```python
from build123d import *

# Parameters (mm, degrees)
SKETCH_1_R          = 3
EXTRUDE_1_DEPTH     = 3
CHAMFER_1_SIZE      = 0.2
SKETCH_2_OUTSIDE_W  = 22.662
SKETCH_2_OUTSIDE_H  = 21.114
SKETCH_2_OUTSIDE_R  = 5
CUT_EXTRUDE_1_DEPTH = 3
CUT_EXTRUDE_1_TAPER = 45
SKETCH_3_OUTSIDE_W  = 22.662
SKETCH_3_OUTSIDE_H  = 21.114
SKETCH_3_OUTSIDE_R  = 5
CUT_EXTRUDE_2_DEPTH = 3
CUT_EXTRUDE_2_TAPER = 45


with BuildPart() as part:
    # Эскиз1 → Бобышка-Вытянуть1 (new body)
    with BuildSketch(Plane.XY):
        Polygon((5.773502692, 0), (2.886751346, 5), (-2.886751346, 5), (-5.773502692, 0), (-2.886751346, -5), (2.886751346, -5), align=None)
        Circle(SKETCH_1_R, mode=Mode.SUBTRACT)
    extrude(amount=EXTRUDE_1_DEPTH)

    # Фаска1
    chamfer_1_edges = [part.edges().sort_by_distance(p)[0] for p in [
        (-3, 0, 0),
        (-3, 0, 3),
    ]]
    chamfer(chamfer_1_edges, length=CHAMFER_1_SIZE)

    # Эскиз2 outside → Вырез-Вытянуть1 (cut)
    with BuildSketch(Plane.XY.offset(3)):
        Rectangle(SKETCH_2_OUTSIDE_W, SKETCH_2_OUTSIDE_H)
        Circle(SKETCH_2_OUTSIDE_R, mode=Mode.SUBTRACT)
    extrude(amount=-CUT_EXTRUDE_1_DEPTH, taper=CUT_EXTRUDE_1_TAPER, mode=Mode.SUBTRACT)

    # Эскиз3 outside → Вырез-Вытянуть2 (cut)
    with BuildSketch(Plane(origin=(0, 0, 0), x_dir=(-1, 0, 0), z_dir=(0, 0, -1))):
        Rectangle(SKETCH_3_OUTSIDE_W, SKETCH_3_OUTSIDE_H)
        Circle(SKETCH_3_OUTSIDE_R, mode=Mode.SUBTRACT)
    extrude(amount=-CUT_EXTRUDE_2_DEPTH, taper=CUT_EXTRUDE_2_TAPER, mode=Mode.SUBTRACT)


solid = part.part
```
Input: part model. Units: mm. Frame: model coordinates. Give positions to 0.01 mm unless a question says otherwise; leave off trailing zeros. Order: outer loops, then holes, each group sorted by start corner. A loop starts at its lowest first (then second) coordinate and runs counter-clockwise, first axis right, second up. Notation, with made-up numbers: M 57.25,31 L 64.25,31 A35 ccw 64.25,68 Z; hole C -3,-38.5 d5. An arc over 180 degrees is marked long. Return JSON: item names as keys, results as strings.
1) Section query B-B on z = 2.5. Output: boundary loops of the cut face in (x, y), and give its area (3 significant figures).
Taken from the geometry:
{"outline": "M -5.48,-0.52 L -3.18,-4.48 A5.5 ccw -2.29,-5 L 2.29,-5 A5.5 ccw 3.18,-4.48 L 5.48,-0.52 A5.5 ccw 5.48,0.52 L 3.18,4.48 A5.5 ccw 2.29,5 L -2.29,5 A5.5 ccw -3.18,4.48 L -5.48,0.52 A5.5 ccw Z; hole C 0,0 d6", "area": "57.5 mm2"}
2) Section query A-A on z = 1.55. Output: boundary loops of the cut face in (x, y), and give its area (3 significant figures).
Taken from the geometry:
{"outline": "M -5.77,0 L -2.89,-5 L 2.89,-5 L 5.77,0 L 2.89,5 L -2.89,5 Z; hole C 0,0 d6", "area": "58.3 mm2"}
3) Contact query for a flat-ended pin moving along its axis: pin 1 (1 mm diameter, centred on y = 2, z = 1, fed in from -X). Output: stop coordinate, or through.
Taken from the geometry:
{"pin 1": "stops at x = -4.91"}
4) Mould query, pull axis Y, two halves, no side actions, for faces 1 (the face through (4.31, -2.535, 1.479)), 2 (the face through (-3, 0, 1)), 3 (the face through (2.583, 4.499, 2.812)). Classes: released by +Y, released by -Y, zero draft, split by the parting line, or undercut.
Taken from the geometry:
{"face 1": "released by -Y", "face 2": "undercut", "face 3": "released by +Y"}
5) Line query: L1, parallel to Y at x = 0, z = 1.1; L2, parallel to X at y = 2.5, z = 0.9; L3, parallel to X at y = 2.75, z = 0.3. Output: solid intervals per line, ascending. Write a range as [from, to].
Taken from the geometry:
{"L1": "y = [-5, -3], [3, 5]", "L2": "x = [-4.33, -1.66], [1.66, 4.33]", "L3": "x = [-4.19, -1.2], [1.2, 4.19]"}
